Here's how the part is built. I have some questions about the finished solid (model axes, mm). A direction names the side the tool comes from. Round coordinates to 2 decimals unless told otherwise and drop trailing zeros. Write each loop counter-clockwise with the first axis right and the second up, starting at its lowest first coordinate (ties: lowest second). Pieces come first, ordered by that corner, then holes. Notation, with made-up numbers: M 47,64 L 90,64 A28 ccw 90,84 Z; hole C 18.5,71 d2. An arc over 180 degrees is marked long. Write item = value, one per line. Start each with the question number.
(1) Will this pin go through, and if not, where does the flat tip stop? pin 1 Ø0.8 at (y, z) = (77.5, 0.5) entering from +X.
(2) I want a section at B-B (x = -36). List the corners of the cut face in (y, z) for me (3 decimals).
(3) I want a section at A-A (y = 14). List the corners of the cut face in (x, z) for me (3 decimals).
(4) I want a section at D-D (y = 32.5). List the corners of the cut face in (x, z) for me, and give its area (3 significant figures).
(5) I want a section at C-C (z = 0.45). List the corners of the cut face in (x, y) for me (3 decimals).
(6) On a 3-axis mill with a long thin cutter (end or side, diameter ignored), from which of +Z, -Z, +X, -X, +Y, -Y can I reach the whole of each face in a straight line? I mean faces 1 (the flat face through (-68, 72, 1)), 2 (the flat face through (-33, 41, 1.5)). Say none if no direction works.
(7) I need wall thicknesses on line 1 along Y through (x, z) = (-36, 0.85) (3 decimals); line 2 along X through (y, z) = (27, 0.3); line 3 along Y through (x, z) = (-37, 1.2). Which ranges of each line are inside material? Lowest first, please.
Autodesk Inventor part; units mm, degrees
ref_plane "YZ Plane" through (0, 0, 0) normal (1, 0, 0) x (0, 1, 0)
ref_plane "XZ Plane" through (0, 0, 0) normal (0, 1, 0) x (-1, 0, 0)
ref_plane "XY Plane" through (0, 0, 0) normal (0, 0, 1) x (1, 0, 0)
sketch "Sketch1" plane through (0, 0, 0) normal (0, 0, 1) x (1, 0, 0)
  line L0 (0, 0) -> (-72, 0)
  circle A0 centre (-72, 68) radius 8 construction
  line L1 (-72, 60) -> (0, 60) construction
  line L2 (-72, 76) -> (-64, 68)
  line L3 (-72, 60) -> (-64, 68)
  line L4 (0, 60) -> (0, 0)
  line L5 (-72, 0) -> (-72, 60)
  line L6 (-72, 76) -> (-72, 80)
  line L7 (0, 76) -> (0, 80)
  line L8 (-72, 80) -> (0, 80)
  line L9 (-72, 76) -> (11.0791, 76) construction
  line L10 (-64, 68) -> (11.3495, 68) construction
  line L11 (-72, 60) -> (22.6598, 60) construction
  circle A1 centre (0, 68) radius 8 construction
  line L12 (0, 60) -> (8, 68)
  line L13 (8, 68) -> (0, 76)
  line L14 (-36, 0) -> (-36, 14) construction
  circle A2 centre (-36, 14) radius 3.075
  point P0 (0, 0)
  point P1 (0, 78)
  point P2 (-72, 78)
  dimension "d0" = 80
  dimension "d2" = 60
  dimension "d3" = 0
  dimension "d4" = 0
  dimension "d5" = 72
  dimension "d8" = 14
  dimension "d9" = 6.15
  dimension "d12" = 36
extrude "Extrusion2" add sketch "Sketch1" along normal blind 1.5
properties part number "MS_RI_black_v3"
Returned:
q1.pin_1 = 0
q2.outline = M 0,0 L 10.925,0 L 10.925,1.5 L 0,1.5 Z; M 17.075,0 L 80,0 L 80,1.5 L 17.075,1.5 Z
q3.outline = M -72,0 L -39.075,0 L -39.075,1.5 L -72,1.5 Z; M -32.925,0 L 0,0 L 0,1.5 L -32.925,1.5 Z
q4.outline = M -72,0 L 0,0 L 0,1.5 L -72,1.5 Z
q4.area = 108 mm²
q5.outline = M -72,0 L 0,0 L 0,60 L 8,68 L 0,76 L 0,80 L -72,80 L -72,76 L -64,68 L -72,60 Z; hole C -36,14 d6.15
q6.face_1 = +Z, -Z, -X
q6.face_2 = +Z, +X, -X, +Y, -Y
q7.line_1 = 0 to 10.925, 17.075 to 80
q7.line_2 = -72 to 0
q7.line_3 = 0 to 11.09, 16.91 to 80
